```python
from build123d import *

# Parameters (mm, degrees)
SKETCH1_W                = 56.2
SKETCH1_H                = 30
BOSS_EXTRUDE1_DEPTH      = 5
SKETCH3_W                = 56.2
SKETCH3_H                = 30
BOSS_EXTRUDE2_DEPTH      = 3
SKETCH4_R                = 1.7
CUT_EXTRUDE2_DEPTH       = 8
SKETCH8_R                = 2.6
CUT_EXTRUDE4_DEPTH       = 4
SKETCH9_W                = 15
SKETCH9_H                = 30
BOSS_EXTRUDE5_DEPTH      = 17
BOSS_EXTRUDE5_DEPTH_BACK = 17
BOSS_EXTRUDE6_DEPTH      = 12
SKETCH11_R               = 2.2
CUT_EXTRUDE5_DEPTH       = 12
BOSS_EXTRUDE7_DEPTH      = 18
CUT_EXTRUDE6_DEPTH       = 18
SKETCH14_R               = 3.25
CUT_EXTRUDE7_DEPTH       = 8


with BuildPart() as part:
    # Sketch1 → Boss-Extrude1 (new body)
    with BuildSketch(Plane.XY):
        with Locations((28.1, -15)):
            Rectangle(SKETCH1_W, SKETCH1_H)
    extrude(amount=BOSS_EXTRUDE1_DEPTH)

    # Sketch3 → Boss-Extrude2 (add)
    with BuildSketch(Plane.XY.offset(5)):
        with Locations((28.1, -15)):
            Rectangle(SKETCH3_W, SKETCH3_H)
    extrude(amount=BOSS_EXTRUDE2_DEPTH)

    # Sketch4 → Cut-Extrude2 (cut)
    with BuildSketch(Plane(origin=(0, 0, 0), x_dir=(-1, 0, 0), z_dir=(0, 0, -1))):
        with Locations((-49.2, -7)):
            Circle(SKETCH4_R)
        with Locations((-7, -7)):
            Circle(SKETCH4_R)
        with Locations((-7, -23)):
            Circle(SKETCH4_R)
        with Locations((-49.2, -23)):
            Circle(SKETCH4_R)
    extrude(amount=-CUT_EXTRUDE2_DEPTH, mode=Mode.SUBTRACT)

    # Sketch8 → Cut-Extrude4 (cut)
    with BuildSketch(Plane(origin=(0, 0, 0), x_dir=(-1, 0, 0), z_dir=(0, 0, -1))):
        with Locations((-49.2, -7)):
            Circle(SKETCH8_R)
        with Locations((-7, -7)):
            Circle(SKETCH8_R)
        with Locations((-7, -23)):
            Circle(SKETCH8_R)
        with Locations((-49.2, -23)):
            Circle(SKETCH8_R)
    extrude(amount=-CUT_EXTRUDE4_DEPTH, mode=Mode.SUBTRACT)

    # Sketch9 → Boss-Extrude5 (add, two sides)
    with BuildSketch(Plane(origin=(28.1, 0, 0), x_dir=(0, 0, -1), z_dir=(1, 0, 0))) as boss_extrude5_sk:
        with Locations((7.5, -15)):
            Rectangle(SKETCH9_W, SKETCH9_H)
    extrude(amount=BOSS_EXTRUDE5_DEPTH)
    extrude(boss_extrude5_sk.sketch, amount=-BOSS_EXTRUDE5_DEPTH_BACK)

    # Sketch10 → Boss-Extrude6 (add)
    with BuildSketch(Plane(origin=(0, 0, 0), x_dir=(1, 0, 0), z_dir=(0, 1, 0))):
        with BuildLine():
            Line((53.1, 15), (3.1, 15))
            ThreePointArc((3.1, 15), (-3.971068, 17.928932), (-6.9, 25))
            Line((-6.9, 25), (-6.9, 70))
            ThreePointArc((-6.9, 70), (-3.971068, 77.071068), (3.1, 80))
            Line((3.1, 80), (53.1, 80))
            ThreePointArc((53.1, 80), (60.171068, 77.071068), (63.1, 70))
            Line((63.1, 70), (63.1, 25))
            ThreePointArc((63.1, 25), (60.171068, 17.928932), (53.1, 15))
        make_face()
    extrude(amount=-BOSS_EXTRUDE6_DEPTH)

    # Sketch11 → Cut-Extrude5 (cut)
    with BuildSketch(Plane(origin=(0, 0, 0), x_dir=(1, 0, 0), z_dir=(0, 1, 0))):
        with Locations((28.1, 70.15)):
            Circle(SKETCH11_R)
        with Locations((53.25, 45)):
            Circle(SKETCH11_R)
        with Locations((28.1, 19.85)):
            Circle(SKETCH11_R)
        with Locations((2.95, 45)):
            Circle(SKETCH11_R)
    extrude(amount=-CUT_EXTRUDE5_DEPTH, mode=Mode.SUBTRACT)

    # Sketch12 → Boss-Extrude7 (add)
    with BuildSketch(Plane(origin=(0, -12, 0), x_dir=(1, 0, 0), z_dir=(0, 1, 0))):
        with BuildLine():
            Line((45.1, 13), (11.1, 13))
            Line((11.1, 13), (11.1, 15))
            Line((11.1, 15), (3.1, 15))
            ThreePointArc((3.1, 15), (-3.971068, 17.928932), (-6.9, 25))
            Line((-6.9, 25), (-6.9, 40))
            Line((-6.9, 40), (-2.494117, 40))
            ThreePointArc((-2.494117, 40), (28.1, 14), (58.694117, 40))
            Line((58.694117, 40), (63.1, 40))
            Line((63.1, 40), (63.1, 25))
            ThreePointArc((63.1, 25), (60.171068, 17.928932), (53.1, 15))
            Line((53.1, 15), (45.1, 15))
            Line((45.1, 15), (45.1, 13))
        make_face()
    extrude(amount=-BOSS_EXTRUDE7_DEPTH)

    # Sketch13 → Cut-Extrude6 (cut)
    with BuildSketch(Plane(origin=(0, -12, 0), x_dir=(1, 0, 0), z_dir=(0, 1, 0))):
        with BuildLine():
            Line((20.28975, 15), (35.91025, 15))
            ThreePointArc((35.91025, 15), (28.1, 14), (20.28975, 15))
        make_face()
    extrude(amount=-CUT_EXTRUDE6_DEPTH, mode=Mode.SUBTRACT)

    # Sketch14 → Cut-Extrude7 (cut)
    with BuildSketch(Plane(origin=(0, 0, 0), x_dir=(1, 0, 0), z_dir=(0, 1, 0))):
        with Locations((28.1, 70.15)):
            Circle(SKETCH14_R)
        with Locations((53.25, 45)):
            Circle(SKETCH14_R)
        with Locations((28.1, 19.85)):
            Circle(SKETCH14_R)
        with Locations((2.95, 45)):
            Circle(SKETCH14_R)
    extrude(amount=-CUT_EXTRUDE7_DEPTH, mode=Mode.SUBTRACT)


solid = part.part
```
Check sheet for the modelled part. Datum: model origin and axes. Units: mm. A direction names the side the tool comes from. Round coordinates to 2 decimals unless told otherwise and drop trailing zeros. Loops run counter-clockwise (first coordinate to the right, second up) from the corner with the lowest first, then second, coordinate; pieces in that order, holes last. Notation, with made-up numbers: (37, 39) - (49, 39) arc R7 cw to (49, 51) - close; hole circle Ø7 at (-4, -37). An arc over 180 degrees is marked (long way). Write item = value, one per line. Start each with the question number.
Q1. Release check for a two-part mould opening along X. For faces 1 (the face through (47.63, -7.65, 5.97)), 2 (the face through (60.25, -14.79, -18.01)), 3 (the face through (61, -21, -40)) record: pulls with the +X half, pulls with the -X half, needs draft (parallel to the pull), parting line crosses it, or undercut.
Q2. Access from +Z, -Z, +X, -X, +Y, -Y to the whole of each face (thin tool, end or side, straight path). Record for faces 4 (the face through (54.75, -3.944, -42.117)), 5 (the face through (11.1, -15, -7)), 6 (the face through (49, -25, 4)), 7 (the face through (51, -15, 0)).
Q3. Section check A-A (x = 28.1). Record the boundary of the cut face in (y, z), plus the area to 3 significant figures.
Q4. Thickness scan on L1, parallel to Z at x = 28.1, y = -2; L2, parallel to Y at x = 7, z = 1; L3, parallel to Y at x = 7, z = 5.7. Record the ranges inside material, lowest first.
Q5. Section check D-D (z = -19.85). Record the boundary of the cut face in (x, y).
Q6. Section check B-B (y = -2). Record the boundary of the cut face in (x, z).
Q7. Depth check by flat-ended pin: P1, Ø6, axis at x = 2.95, z = -45, coming from the -Y side; P2, Ø5, axis at x = 1.5, z = -46.5, coming from the +Y side; P3, Ø9, axis at y = -16, z = 4, coming from the +X side; P4, Ø5, axis at x = -4, y = -25, coming from the -Z side. Enter the tip coordinate at first touch or a pass-through.
Q8. Section check C-C (y = -23). Count the separate pieces of the cut face and the enclosed holes in it, plus the area to 3 significant figures.
Derived:
q1.face_1 = undercut
q1.face_2 = pulls with the +X half
q1.face_3 = needs draft
q2.face_4 = +Y
q2.face_5 = -X, +Y, -Y
q2.face_6 = none
q2.face_7 = +X, +Y, -Y
q3.outline = (-30, -14) - (-12, -14) - (-12, -17.65) - (-8, -17.65) - (-8, -16.6) - (0, -16.6) - (0, 8) - (-30, 8) - close; (-12, -80) - (0, -80) - (0, -73.4) - (-8, -73.4) - (-8, -72.35) - (-12, -72.35) - close; (-12, -67.95) - (-8, -67.95) - (-8, -66.9) - (0, -66.9) - (0, -23.1) - (-8, -23.1) - (-8, -22.05) - (-12, -22.05) - close
q3.area = 1,310 mm^2
q4.L1 = -80 to -73.4, -66.9 to -23.1, -16.6 to 8
q4.L2 = -30 to -25.6, -20.4 to -9.6, -4.4 to 0
q4.L3 = -30 to -24.7, -21.3 to -8.7, -5.3 to 0
q5.outline = (-5.47, -30) - (9.98, -30) - (9.98, -12) - (25.9, -12) - (25.9, -8) - (24.85, -8) - (24.85, 0) - (-5.47, 0) - close; (30.3, -12) - (46.22, -12) - (46.22, -30) - (61.67, -30) - (61.67, 0) - (31.35, 0) - (31.35, -8) - (30.3, -8) - close
q6.outline = (-6.9, -70) arc R10 ccw to (3.1, -80) - (53.1, -80) arc R10 ccw to (63.1, -70) - (63.1, -25) arc R10 ccw to (53.1, -15) - (45.1, -15) - (45.1, 0) - (56.2, 0) - (56.2, 8) - (0, 8) - (0, 0) - (11.1, 0) - (11.1, -15) - (3.1, -15) arc R10 ccw to (-6.9, -25) - close; hole circle Ø6.5 at (2.95, -45); hole circle Ø6.5 at (28.1, -70.15); hole circle Ø6.5 at (28.1, -19.85); hole circle Ø6.5 at (53.25, -45)
q7.P1 = -12
q7.P2 = 0
q7.P3 = 56.2
q7.P4 = -40
q8.separate_pieces = 3
q8.enclosed_holes = 0
q8.area = 1,400 mm^2
